Here's how the part is built. I have some questions about the finished solid (model axes, mm). A direction names the side the tool comes from. Coordinates: 2 decimals unless noted, no trailing zeros. Write each loop counter-clockwise with the first axis right and the second up, starting at its lowest first coordinate (ties: lowest second). Pieces come first, ordered by that corner, then holes.
```python
from build123d import *

# Parameters (mm, degrees)
F1_DEPTH = 29
F2_W     = 36
F2_H     = 11
F3_DEPTH = 63.5


with BuildPart() as f1:
    # F0 (on Front) → F1 (new body, symmetric)
    with BuildSketch(Plane.XZ):
        with BuildLine():
            Line((-52.5, 9), (-52.5, 0))
            Line((-52.5, 0), (52.5, 0))
            Line((52.5, 0), (52.5, 9))
            Line((52.5, 9), (63.5, 9))
            ThreePointArc((63.5, 9), (55.006097, 29.506097), (34.5, 38))
            Line((34.5, 38), (-34.5, 38))
            ThreePointArc((-34.5, 38), (-55.006097, 29.506097), (-63.5, 9))
            Line((-63.5, 9), (-52.5, 9))
        make_face()
    extrude(amount=F1_DEPTH, both=True)

    # F2 (on Right) → F3 (cut, symmetric)
    with BuildSketch(Plane.YZ):
        with Locations((0, 32.5)):
            Rectangle(F2_W, F2_H)
    extrude(amount=F3_DEPTH, both=True, mode=Mode.SUBTRACT)


solid = f1.part
```
1) Imagine slicing it at D-D on z = 25. Please give me the cut outline in (x, y), then the cut area to 3 significant figures.
Values follow:
outline: (-58.69, -29) - (58.69, -29) - (58.69, 29) - (-58.69, 29) - close
area: 6,810 mm2
2) I need wall thicknesses on probe 1 along Y at (x, z) = (-46, 32); probe 2 along Z at (x, y) = (-2.5, -2.5); probe 3 along X at (y, z) = (-8.5, 6). Which ranges of each line are inside material? Lowest first, please.
Values follow:
probe 1: y = -29 to -18, 18 to 29
probe 2: z = 0 to 27
probe 3: x = -52.5 to 52.5
3) Imagine slicing it at A-A on x = -8. Please give me the cut outline in (y, z), then the cut area to 3 significant figures.
Values follow:
outline: (-29, 0) - (29, 0) - (29, 38) - (18, 38) - (18, 27) - (-18, 27) - (-18, 38) - (-29, 38) - close
area: 1,810 mm2
4) Will these pins go through, and if not, where does the flat tip stop? pin 1 (2.5 mm diameter, centred on y = -9, z = 3.5, fed in from +X); pin 2 (11 mm diameter, centred on x = 22, y = -6, fed in from +Z); pin 3 (9 mm diameter, centred on x = 57.5, y = 2, fed in from -Z).
Values follow:
pin 1: stops at x = 52.5
pin 2: stops at z = 27
pin 3: stops at z = 9
5) Imagine slicing it at C-C on z = 5.5. Please give me the cut outline in (x, y), then the cut area to 3 significant figures.
Values follow:
outline: (-52.5, -29) - (52.5, -29) - (52.5, 29) - (-52.5, 29) - close
area: 6,090 mm2
6) On a 3-axis mill with a long thin cutter (end or side, diameter ignored), from which of +Z, -Z, +X, -X, +Y, -Y can I reach the whole of each face in a straight line? I mean faces 5 (the face through (1, 0, 27)), 6 (the face through (-52.5, 0, 5)), 7 (the face through (52.5, 0, 4)). Say none if no direction works.
Values follow:
face 5: +Z, +X, -X
face 6: -Z, -X, +Y, -Y
face 7: -Z, +X, +Y, -Y
7) We'd pull the mould along Y, two halves only. Please class faces 1 (the face through (1, -18, 32)), 2 (the face through (58, 0, 9)), 3 (the face through (1, 18, 32)), 4 (the face through (-1, -29, 19)): pulls with the +Y half, pulls with the -Y half, needs draft (parallel to the pull), parting line crosses it, or undercut.
Values follow:
face 1: undercut
face 2: needs draft
face 3: undercut
face 4: pulls with the -Y half
8) Imagine slicing it at B-B on y = -5.5. Please give me the cut outline in (x, z).
Values follow:
outline: (-63.5, 9) - (-52.5, 9) - (-52.5, 0) - (52.5, 0) - (52.5, 9) - (63.5, 9) arc R29 ccw to (57.24, 27) - (-57.24, 27) arc R29 ccw to start
